Could you check a few things on this model? Use its own coordinates, in mm. Face numbers are marked on the shaded views. A direction names the side the tool comes from. Round coordinates to 2 decimals unless told otherwise and drop trailing zeros. Write each loop counter-clockwise with the first axis right and the second up, starting at its lowest first coordinate (ties: lowest second). Pieces come first, ordered by that corner, then holes. Notation, with made-up numbers: (-14, 73) -> (13, 73) arc R16 ccw to (13, 85) -> close; hole circle Ø4 at (42, -10). An arc over 180 degrees is marked (long way). Answer as CSV lines item,"result". Start each with the question number.
Q1. Imagine slicing it at A-A on z = -190. Please give me the cut outline in (x, y), and give its area (3 significant figures).
Q2. Imagine slicing it at C-C on x = -687. Please give me the cut outline in (y, z).
Q3. If we mould it in two halves opening along X, with no side actions, what happens to the marked faces 4, 5, 6 and 7? For each: pulls with the +X half, pulls with the -X half, needs draft (parallel to the pull), parting line crosses it, or undercut.
Q4. Will these pins go through, and if not, where does the flat tip stop? pin 1 Ø4 at (y, z) = (-41, -332.5) entering from -X; pin 2 Ø1 at (y, z) = (-137.5, -345) entering from +X.
Q5. For the marked faces 1, 2 and 3, which set-ups out of +Z, -Z, +X, -X, +Y, -Y let a thin tool reach every point of the face, with its end or its side?
Q6. Imagine slicing it at B-B on y = -147.5. Please give me the cut outline in (x, z), and give its area (3 significant figures).
Q7. If I drill on line 1 (X direction, y = 10.5, z = -500); line 2 (Z direction, x = 611.5, y = -19.5), over which ranges is the centre line in solid material (lowest first)? Write a range as [from, to].
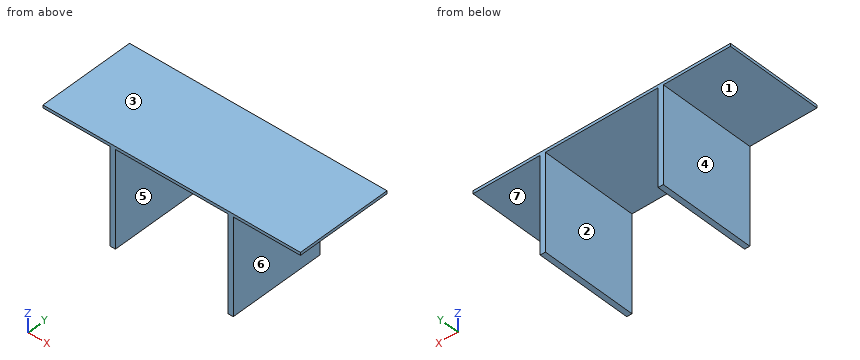
from build123d import *

# Parameters (mm, degrees)
F0_W     = 32.559776
F0_H     = 600
F0_W_2   = 417.440581
F0_W_3   = 32.559419
F0_W_4   = 417.440224
F0_W_5   = 700
F1_DEPTH = 18
F2_DEPTH = 600


with BuildPart() as f1:
    # F0 (on Top) → F1 (new body)
    with BuildSketch(Plane.XY):
        with Locations((366.279888, 0)):
            Rectangle(F0_W, F0_H)
        with Locations((-591.279709, 0)):
            Rectangle(F0_W_2, F0_H)
        with Locations((-366.279709, 0)):
            Rectangle(F0_W_3, F0_H)
        with Locations((591.279888, 0)):
            Rectangle(F0_W_4, F0_H)
        Rectangle(F0_W_5, F0_H)
    extrude(amount=F1_DEPTH)

    # F0 (on Top) → F2 (join)
    with BuildSketch(Plane.XY):
        with Locations((-366.279709, 0)):
            Rectangle(F0_W_3, F0_H)
        with Locations((366.279888, 0)):
            Rectangle(F0_W, F0_H)
    extrude(amount=-F2_DEPTH)


solid = f1.part
Checks:
1,outline,"(-382.56, -300) -> (-350, -300) -> (-350, 300) -> (-382.56, 300) -> close; (350, -300) -> (382.56, -300) -> (382.56, 300) -> (350, 300) -> close"
1,area,"39,100 mm^2"
2,outline,"(-300, 0) -> (300, 0) -> (300, 18) -> (-300, 18) -> close"
3,face 4,"pulls with the -X half"
3,face 5,"undercut"
3,face 6,"pulls with the +X half"
3,face 7,"needs draft"
4,pin 1,"x = -382.56"
4,pin 2,"x = 382.56"
5,face 1,"-Z, -X, +Y, -Y"
5,face 2,"-Z, +Y, -Y"
5,face 3,"+Z, +X, -X, +Y, -Y"
6,outline,"(-800, 0) -> (-382.56, 0) -> (-382.56, -600) -> (-350, -600) -> (-350, 0) -> (350, 0) -> (350, -600) -> (382.56, -600) -> (382.56, 0) -> (800, 0) -> (800, 18) -> (-800, 18) -> close"
6,area,"67,900 mm^2"
7,line 1,"[-382.56, -350], [350, 382.56]"
7,line 2,"[0, 18]"
